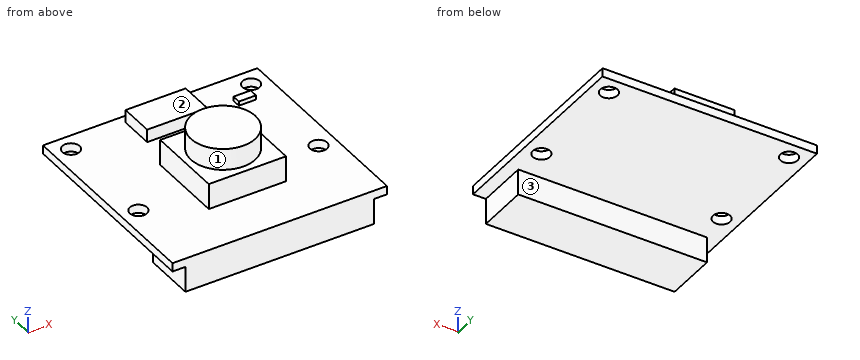
from build123d import *

# Parameters (mm, degrees)
CROQUIS1_W              = 25
CROQUIS1_H              = 24
CROQUIS1_R              = 1
CROQUIS1_W_2            = 2
CROQUIS1_H_2            = 1
CROQUIS1_W_3            = 7
CROQUIS1_H_3            = 4
CROQUIS1_W_4            = 9
CROQUIS1_H_4            = 9
SALIENTE_EXTRUIR1_DEPTH = 1
CROQUIS1_3_W            = 2
CROQUIS1_3_H            = 1
SALIENTE_EXTRUIR2_DEPTH = 1.5
CROQUIS1_4_W            = 7
CROQUIS1_4_H            = 4
SALIENTE_EXTRUIR3_DEPTH = 2.5
CROQUIS1_5_W            = 9
CROQUIS1_5_H            = 9
SALIENTE_EXTRUIR4_DEPTH = 4
CROQUIS3_R              = 3.75
SALIENTE_EXTRUIR5_DEPTH = 2.5
CROQUIS4_W              = 22
CROQUIS4_H              = 6
SALIENTE_EXTRUIR6_DEPTH = 3
SCALE1_SCALE            = 1.3


with BuildPart() as part:
    # Croquis1 → Saliente-Extruir1 (new body)
    # profile 1 of 4: a face of its own
    with BuildSketch(Plane.XY):
        with Locations((0, 1.5)):
            Rectangle(CROQUIS1_W, CROQUIS1_H)
        with Locations((10.5, -1)):
            Circle(CROQUIS1_R, mode=Mode.SUBTRACT)
        with Locations((-10.5, -1)):
            Circle(CROQUIS1_R, mode=Mode.SUBTRACT)
        with Locations((10.5, 11.5)):
            Circle(CROQUIS1_R, mode=Mode.SUBTRACT)
        with Locations((-10.5, 11.5)):
            Circle(CROQUIS1_R, mode=Mode.SUBTRACT)
        with Locations((8.5, 9.5)):
            Rectangle(CROQUIS1_W_2, CROQUIS1_H_2, mode=Mode.SUBTRACT)
        with Locations((0, 10.5)):
            Rectangle(CROQUIS1_W_3, CROQUIS1_H_3, mode=Mode.SUBTRACT)
        Rectangle(CROQUIS1_W_4, CROQUIS1_H_4, mode=Mode.SUBTRACT)
    # profile 2 of 4: a face of its own
    with BuildSketch(Plane.XY):
        Rectangle(CROQUIS1_W_4, CROQUIS1_H_4)
    # profile 3 of 4: a face of its own
    with BuildSketch(Plane.XY):
        with Locations((0, 10.5)):
            Rectangle(CROQUIS1_W_3, CROQUIS1_H_3)
    # profile 4 of 4: a face of its own
    with BuildSketch(Plane.XY):
        with Locations((8.5, 9.5)):
            Rectangle(CROQUIS1_W_2, CROQUIS1_H_2)
    extrude(amount=SALIENTE_EXTRUIR1_DEPTH)

    # Croquis1_3 → Saliente-Extruir2 (add)
    with BuildSketch(Plane.XY):
        with Locations((8.5, 9.5)):
            Rectangle(CROQUIS1_3_W, CROQUIS1_3_H)
    extrude(amount=SALIENTE_EXTRUIR2_DEPTH)

    # Croquis1_4 → Saliente-Extruir3 (add)
    with BuildSketch(Plane.XY):
        with Locations((0, 10.5)):
            Rectangle(CROQUIS1_4_W, CROQUIS1_4_H)
    extrude(amount=SALIENTE_EXTRUIR3_DEPTH)

    # Croquis1_5 → Saliente-Extruir4 (add)
    with BuildSketch(Plane.XY):
        Rectangle(CROQUIS1_5_W, CROQUIS1_5_H)
    extrude(amount=SALIENTE_EXTRUIR4_DEPTH)

    # Croquis3 → Saliente-Extruir5 (add)
    with BuildSketch(Plane.XY.offset(4)):
        Circle(CROQUIS3_R)
    extrude(amount=SALIENTE_EXTRUIR5_DEPTH)

    # Croquis4 → Saliente-Extruir6 (add)
    with BuildSketch(Plane(origin=(0, 0, 0), x_dir=(-1, 0, 0), z_dir=(0, 0, -1))):
        with Locations((0, -7.5)):
            Rectangle(CROQUIS4_W, CROQUIS4_H)
    extrude(amount=SALIENTE_EXTRUIR6_DEPTH)


with BuildPart() as part_1:
    # Scale1: scaled about (0, 0, 0)
    add(part.part.scale(SCALE1_SCALE))


solid = part_1.part
Model file for the job. Use its own axes, mm. Face numbers are marked on the shaded views. A direction names the side the tool comes from. Give positions to 0.01 mm unless a question says otherwise; leave off trailing zeros. Write each loop counter-clockwise with the first axis right and the second up, starting at its lowest first coordinate (ties: lowest second). Pieces come first, ordered by that corner, then holes. Notation, with made-up numbers: M 3.5,22 L 16.5,22 A23 cw 16.5,44 Z; hole C 0.5,80 d1. An arc over 180 degrees is marked long. One line per item, written item: value. Start each with the question number.
Q1. Saw through at C-C, the plane y = -9.5. Write the cut outline in (x, z).
Q2. Probe probe 1 along Y at (x, z) = (-13.65, 0.5); probe 2 along Y at (x, z) = (3, -3); probe 3 along Z at (x, y) = (-6, 9.5). List the from-to ranges inside material, lowest first. Write a range as [from, to].
Q3. Drop flat-ended pins along their axis: pin 1 Ø1.6 at (x, z) = (-0.5, 2.5) entering from -Y; pin 2 Ø0.6 at (y, z) = (13.5, 2) entering from -X; pin 3 Ø5.5 at (x, y) = (-0.5, 13.5) entering from +Z. Give the stop position or say it passes through.
Q4. 3-axis set-ups, long thin cutter, end or side, ignore diameter. For the marked faces 1, 2 and 3: which of +Z, -Z, +X, -X, +Y, -Y reach the whole face in a straight line?
Q5. Saw through at B-B, the plane x = 13.65. Write the cut outline in (y, z).
Q6. Saw through at D-D, the plane x = 0. Write the cut outline in (y, z) (3 decimals).
Q7. Saw through at A-A, the plane y = 14.95. Write the cut outline in (x, z), plus the area to 3 significant figures.
Output values:
1. outline: M -16.25,0 L -14.3,0 L -14.3,-3.9 L 14.3,-3.9 L 14.3,0 L 16.25,0 L 16.25,1.3 L -16.25,1.3 Z
2. probe 1: y = [-13.65, -2.6], [0, 13.65], [16.25, 17.55]
2. probe 2: y = [-13.65, -5.85]
2. probe 3: z = [0, 1.3]
3. pin 1: stops at y = -5.85
3. pin 2: stops at x = -4.55
3. pin 3: stops at z = 3.25
4. face 1: +Z
4. face 2: +Z, +X, -X, +Y
4. face 3: -Z, +X, -X, +Y
5. outline: M -13.65,-3.9 L -5.85,-3.9 L -5.85,0 L -2.6,0 L -2.6,1.3 L -13.65,1.3 Z; M 0,0 L 13.65,0 L 13.65,1.3 L 0,1.3 Z; M 16.25,0 L 17.55,0 L 17.55,1.3 L 16.25,1.3 Z
6. outline: M -13.65,-3.9 L -5.85,-3.9 L -5.85,0 L 17.55,0 L 17.55,1.3 L 16.25,1.3 L 16.25,3.25 L 11.05,3.25 L 11.05,1.3 L 5.85,1.3 L 5.85,5.2 L 4.875,5.2 L 4.875,8.45 L -4.875,8.45 L -4.875,5.2 L -5.85,5.2 L -5.85,1.3 L -13.65,1.3 Z
7. outline: M -16.25,0 L -14.95,0 L -14.95,1.3 L -16.25,1.3 Z; M -12.35,0 L 12.35,0 L 12.35,1.3 L 4.55,1.3 L 4.55,3.25 L -4.55,3.25 L -4.55,1.3 L -12.35,1.3 Z; M 14.95,0 L 16.25,0 L 16.25,1.3 L 14.95,1.3 Z
7. area: 53.2 mm²
